from build123d import *

# Parameters (mm, degrees)
SKETCH1_W           = 127
SKETCH1_H           = 152.4
BOSS_EXTRUDE1_DEPTH = 50.8
CUT_EXTRUDE1_DEPTH  = 156.939365922
CUT_EXTRUDE2_DEPTH  = 186.205309499
SKETCH6_R           = 10.16
CUT_EXTRUDE3_DEPTH  = 139.062227017
SKETCH7_R           = 12.7
CUT_EXTRUDE4_DEPTH  = 152.108237347


with BuildPart() as part:
    # Sketch1 → Boss-Extrude1 (new body)
    with BuildSketch(Plane(origin=(0, 0, 0), x_dir=(1, 0, 0), z_dir=(0, 1, 0))):
        Rectangle(SKETCH1_W, SKETCH1_H)
    extrude(amount=BOSS_EXTRUDE1_DEPTH)

    # Sketch3 → Cut-Extrude1 (cut, through all)
    with BuildSketch(Plane(origin=(47.501298701, 59.376623377, 15.833766234), x_dir=(0.7911852033335974, -0.5909267078840147, -0.1575804554357373), z_dir=(0.6115766297251508, 0.7644707871564383, 0.20385887657505028))):
        Polygon((-11.882551218, -60.537839749), (20.221183651, 13.089262648), (20.221183651, -65.773544809), align=None)
    extrude(amount=CUT_EXTRUDE1_DEPTH, mode=Mode.SUBTRACT)

    # Sketch4 → Cut-Extrude2 (cut, through all)
    with BuildSketch(Plane(origin=(55.033333333, 55.033333333, -55.033333333), x_dir=(0.816496580927726, -0.40824829046386363, 0.40824829046386246), z_dir=(0.5773502691896258, 0.577350269189627, -0.5773502691896246))):
        Polygon((-20.739013156, 17.960512242), (10.369506578, 35.921024484), (10.369506578, 0), align=None)
    extrude(amount=CUT_EXTRUDE2_DEPTH, mode=Mode.SUBTRACT)

    # Sketch6 → Cut-Extrude3 (cut, through all)
    with BuildSketch(Plane(origin=(-30.799022248, 66.048716355, 0), x_dir=(0, 0, 1), z_dir=(-0.4226182617407003, 0.9063077870366496, 0))):
        with Locations(Location((50.8, -13.06131899, 0), (0, 0, 270))):
            Circle(SKETCH6_R)
    extrude(amount=-CUT_EXTRUDE3_DEPTH, mode=Mode.SUBTRACT)

    # Sketch7 → Cut-Extrude4 (cut, through all)
    with BuildSketch(Plane(origin=(0, 71.095567884, -41.047045256), x_dir=(-1, 0, 0), z_dir=(0, 0.866025403784438, -0.500000000000001))):
        with Locations(Location((-12.7, -10.208864232, 0), (0, 0, 270))):
            Circle(SKETCH7_R)
    extrude(amount=-CUT_EXTRUDE4_DEPTH, mode=Mode.SUBTRACT)


solid = part.part
Geometry check sheet. Reference: the model listing, model coordinates, mm. Round coordinates to 2 decimals unless told otherwise and drop trailing zeros. Loops run counter-clockwise (first coordinate to the right, second up) from the corner with the lowest first, then second, coordinate; pieces in that order, holes last.
Item 1: Cross-section at A-A on x = 8.5. Record the boundary of the cut face in (y, z), then the cut area to 3 significant figures.
Item 2: Thickness scan on line 1 (Z direction, x = -21, y = 13); line 2 (Z direction, x = -19, y = 19); line 3 (X direction, y = 48, z = 43.5). Record the ranges inside material, lowest first.
Item 3: Mould release check, pull along Z, two halves, no side actions. Record for faces 1 (the flat face through (53.8, 42.8, -68.5)), 2 (the flat face through (-1, 50.8, -1)), 3 (the cylindrical face through (1.991, 22.301, -32.547)): pulls with the +Z half, pulls with the -Z half, needs draft (parallel to the pull), parting line crosses it, or undercut.
Item 4: Cross-section at C-C on y = 46. Count the separate pieces of the cut face and the enclosed holes in it, then the cut area to 3 significant figures.
Item 5: Cross-section at B-B on x = 52.5. Record the boundary of the cut face in (y, z).
Answer sheet:
1. outline: (0, -76.2) - (50.8, -76.2) - (50.8, -54.96) - (0, -25.63) - close; (0, 2.05) - (50.8, -27.28) - (50.8, 76.2) - (0, 76.2) - close
1. area: 6,340 mm2
2. line 1: z = -76.2 to 40.65, 60.95 to 76.2
2. line 2: z = -76.2 to 41.41, 60.19 to 76.2
2. line 3: x = -63.5 to -44.59, -29 to 52.5
3. face 1: pulls with the -Z half
3. face 2: needs draft
3. face 3: undercut
4. separate pieces: 1
4. enclosed holes: 2
4. area: 17,600 mm2
5. outline: (0, -76.2) - (36.4, -76.2) - (50.8, -61.8) - (50.8, 33) - (39.28, 76.2) - (0, 76.2) - close
